```python
from build123d import *

# Parameters (mm, degrees)
F0_W             = 150
F0_H             = 90
F1_DEPTH         = 20
F2_R             = 5.5
F3_DEPTH         = 20.001
F4_W             = 2
F4_H             = 28
F5_DEPTH         = 150.001
F6_W             = 150
F6_H             = 124
F6_R             = 30
F7_DEPTH         = 20
F9_DEPTH         = 20.001
F11_W            = 150
F11_H            = 20
F12_DEPTH        = 20
F13_R            = 6
F14_DEPTH        = 20.001
F15_W            = 150
F15_H            = 18
F16_DEPTH        = 20
F17_R            = 52
F17_R_2          = 30
F18_DEPTH        = 20
F20_R            = 62.5
F20_R_2          = 52
F21_DEPTH        = 10
F22_R            = 3.4
F23_DEPTH        = 20.001
F23_COPIES_COUNT = 3
F24_R            = 2.5
F25_DEPTH        = 20.001
F25_COPIES_COUNT = 3


# Not quite as in the source:
# - a pattern or mirror of a feature is missing from the dataset's text; its kind, count and spacing are read off the source's solid


with BuildPart() as f1:
    # F0 (on Front) → F1 (new body)
    with BuildSketch(Plane.XZ):
        with Locations((0, -15)):
            Rectangle(F0_W, F0_H)
    extrude(amount=F1_DEPTH)

    # F2 (on face) → F3 (cut, through all)
    with BuildSketch(Plane.XZ.offset(20)):
        with Locations((-60, -45)):
            Circle(F2_R)
        with Locations((60, -45)):
            Circle(F2_R)
    extrude(amount=-F3_DEPTH, mode=Mode.SUBTRACT)

    # F4 (on face) → F5 (cut, through all)
    with BuildSketch(Plane(origin=(-75, 0, 0), x_dir=(0, -1, 0), z_dir=(-1, 0, 0))):
        with Locations((19, -9.5)):
            Rectangle(F4_W, F4_H)
    extrude(amount=-F5_DEPTH, mode=Mode.SUBTRACT)

    # F6 (on face) → F7 (join)
    with BuildSketch(Plane(origin=(0, 0, 0), x_dir=(-1, 0, 0), z_dir=(0, 1, 0))):
        with Locations((0, 92)):
            Rectangle(F6_W, F6_H)
        with Locations((0, 97)):
            Circle(F6_R, mode=Mode.SUBTRACT)
    extrude(amount=-F7_DEPTH)

    # F8 (on face) → F9 (cut, through all)
    with BuildSketch(Plane(origin=(0, 0, 0), x_dir=(-1, 0, 0), z_dir=(0, 1, 0))):
        with BuildLine():
            ThreePointArc((-75, -39.6602540378), (-71.3397459622, -36), (-70, -31))
            ThreePointArc((-70, -31), (-71.3397459622, -26), (-75, -22.3397459622))
            Line((-75, -22.3397459622), (-75, -39.6602540378))
        make_face()
        with BuildLine():
            Line((-75, -39.6602540378), (-75, -22.3397459622))
            ThreePointArc((-75, -22.3397459622), (-90, -31), (-75, -39.6602540378))
        make_face()
        with BuildLine():
            Line((75, -39.6602540378), (75, -22.3397459622))
            ThreePointArc((75, -22.3397459622), (70, -31), (75, -39.6602540378))
        make_face()
        with BuildLine():
            ThreePointArc((90, -31), (85, -22.3397459622), (75, -22.3397459622))
            Line((75, -22.3397459622), (75, -39.6602540378))
            ThreePointArc((75, -39.6602540378), (85, -39.6602540378), (90, -31))
        make_face()
    extrude(amount=-F9_DEPTH, mode=Mode.SUBTRACT)

    # F11 (on face) → F12 (join)
    with BuildSketch(Plane(origin=(0, 0, 0), x_dir=(-1, 0, 0), z_dir=(0, 1, 0))):
        with Locations((0, -70)):
            Rectangle(F11_W, F11_H)
    extrude(amount=-F12_DEPTH)

    # F13 (on face) → F14 (cut, through all)
    with BuildSketch(Plane(origin=(0, 0, 0), x_dir=(-1, 0, 0), z_dir=(0, 1, 0))):
        with Locations((0, -57)):
            Circle(F13_R)
    extrude(amount=-F14_DEPTH, mode=Mode.SUBTRACT)

    # F15 (on face) → F16 (join)
    with BuildSketch(Plane.XZ.offset(20)):
        with Locations((0, 163)):
            Rectangle(F15_W, F15_H)
    extrude(amount=-F16_DEPTH)

    # F17 (on face) → F18 (cut)
    with BuildSketch(Plane(origin=(0, 0, 0), x_dir=(-1, 0, 0), z_dir=(0, 1, 0))):
        with Locations((0, 97)):
            Circle(F17_R)
        with Locations((0, 97)):
            Circle(F17_R_2, mode=Mode.SUBTRACT)
    extrude(amount=-F18_DEPTH, mode=Mode.SUBTRACT)

    # F20 (on face) → F21 (cut)
    with BuildSketch(Plane.XZ.offset(20)):
        with Locations((0, 97)):
            Circle(F20_R)
        with Locations((0, 97)):
            Circle(F20_R_2, mode=Mode.SUBTRACT)
    extrude(amount=-F21_DEPTH, mode=Mode.SUBTRACT)

    # F22 (on face) → F23 (cut, through all)
    with BuildSketch(Plane.XZ.offset(20)):
        with Locations((0, 22)):
            Circle(F22_R)
    f23 = extrude(amount=-F23_DEPTH, mode=Mode.SUBTRACT)

    # F23_copies: F23 ×3 about axis
    f23_copies_axis = Axis((0, 0, 97), (0, 1, 0))
    for i in range(1, F23_COPIES_COUNT):
        add(f23.rotate(f23_copies_axis, i * 360 / F23_COPIES_COUNT), mode=Mode.SUBTRACT)

    # F24 (on face) → F25 (cut, through all)
    with BuildSketch(Plane(origin=(0, 0, 0), x_dir=(-1, 0, 0), z_dir=(0, 1, 0))):
        with Locations((0, 156)):
            Circle(F24_R)
    f25 = extrude(amount=-F25_DEPTH, mode=Mode.SUBTRACT)

    # F25_copies: F25 ×3 about axis
    f25_copies_axis = Axis((0, 0, 97), (0, 1, 0))
    for i in range(1, F25_COPIES_COUNT):
        add(f25.rotate(f25_copies_axis, i * 360 / F25_COPIES_COUNT), mode=Mode.SUBTRACT)


solid = f1.part
```
Geometry: final body of the model. Coordinates: model frame, mm. A direction names the side the tool comes from. Coordinates: 2 decimals unless noted, no trailing zeros. Order: outer loops, then holes, each group sorted by start corner. A loop starts at its lowest first (then second) coordinate and runs counter-clockwise, first axis right, second up. Notation, with made-up numbers: (12.5, 11) -> (20.5, 11) arc R16 ccw to (20.5, 17) -> close; hole circle Ø5 at (-13, 69). An arc over 180 degrees is marked (long way). Write item = value, one per line.
(1) Cut plane B-B on z = 97. Return loops of the section in (x, y), plus the area to 3 significant figures.
Solved:
outline = (-75, -20) -> (-62.5, -20) -> (-62.5, -10) -> (-52, -10) -> (-52, 0) -> (-75, 0) -> close; (52, -10) -> (62.5, -10) -> (62.5, -20) -> (75, -20) -> (75, 0) -> (52, 0) -> close
area = 710 mm²
(2) Cut plane C-C on z = 135. Return loops of the section in (x, y).
Solved:
outline = (-75, -20) -> (-68.31, -20) -> (-68.31, 0) -> (-75, 0) -> close; (-61.59, -20) -> (-49.62, -20) -> (-49.62, -10) -> (-35.5, -10) -> (-35.5, 0) -> (-61.59, 0) -> close; (35.5, -10) -> (49.62, -10) -> (49.62, -20) -> (61.59, -20) -> (61.59, 0) -> (35.5, 0) -> close; (68.31, -20) -> (75, -20) -> (75, 0) -> (68.31, 0) -> close
(3) Line query: line 1 (Z direction, x = 0, y = -14.25); line 2 (Z direction, x = 0.5, y = -2); line 3 (Z direction, x = 0, y = -4.25). Output: solid intervals per line, ascending.
Solved:
line_1 = -80 to -63, -51 to 18.6, 25.4 to 34.5, 159.5 to 172
line_2 = -80 to -62.98, -51.02 to 18.64, 25.36 to 45, 149 to 153.55, 158.45 to 172
line_3 = -80 to -63, -51 to 18.6, 25.4 to 45, 149 to 153.5, 158.5 to 172
(4) Pin query (flat end, axial travel): pin 1 Ø8 at (x, z) = (-64.95, 134.5) entering from +Y; pin 2 Ø6 at (x, z) = (-21.5, 51.5) entering from -Y. Return the tip coordinate at first contact, or that it passes through.
Solved:
pin_1 = 0
pin_2 = -10
(5) Cut plane D-D on y = -14. Return loops of the section in (x, z).
Solved:
outline = (-75, -80) -> (75, -80) -> (75, -39.66) arc R10 cw to (75, -22.34) -> (75, 172) -> (-75, 172) -> (-75, -22.34) arc R10 cw to (-75, -39.66) -> close; hole circle Ø6.8 at (-64.95, 134.5); hole circle Ø11 at (-60, -45); hole circle Ø125 at (0, 97); hole circle Ø12 at (0, -57); hole circle Ø6.8 at (0, 22); hole circle Ø11 at (60, -45); hole circle Ø6.8 at (64.95, 134.5)
(6) Cut plane A-A on x = 0. Return loops of the section in (y, z).
Solved:
outline = (-20, -80) -> (0, -80) -> (0, -63) -> (-20, -63) -> close; (-20, -51) -> (0, -51) -> (0, 18.6) -> (-20, 18.6) -> (-20, 4.5) -> (-18, 4.5) -> (-18, -23.5) -> (-20, -23.5) -> close; (-20, 25.4) -> (0, 25.4) -> (0, 45) -> (-10, 45) -> (-10, 34.5) -> (-20, 34.5) -> close; (-20, 159.5) -> (-10, 159.5) -> (-10, 158.5) -> (0, 158.5) -> (0, 172) -> (-20, 172) -> close; (-10, 149) -> (0, 149) -> (0, 153.5) -> (-10, 153.5) -> close
(7) Access query for faces 1 (the cylindrical face through (-13.549, -15.07, 35.986)), 2 (the cylindrical face through (54.505, -10.14, -44.758)). Directions: +Z, -Z, +X, -X, +Y, -Y. A direction counts if a zero-diameter tool reaches every point of the face in a straight line with its end or side. Return the directions, or none.
Solved:
face_1 = -Y
face_2 = +Y, -Y
